Geometry check sheet. Reference: drawing and pictorial views, mm from the part's lowest x, y, z. Give positions to 0.01 mm unless a question says otherwise; leave off trailing zeros. Write each loop counter-clockwise with the first axis right and the second up, starting at its lowest first coordinate (ties: lowest second). Pieces come first, ordered by that corner, then holes. Notation, with made-up numbers: (-27.5, 67) -> (19.5, 67) arc R27 cw to (19.5, 95) -> close; hole circle Ø7 at (22.5, 71.5). An arc over 180 degrees is marked (long way). Return JSON: item names as keys, results as strings.
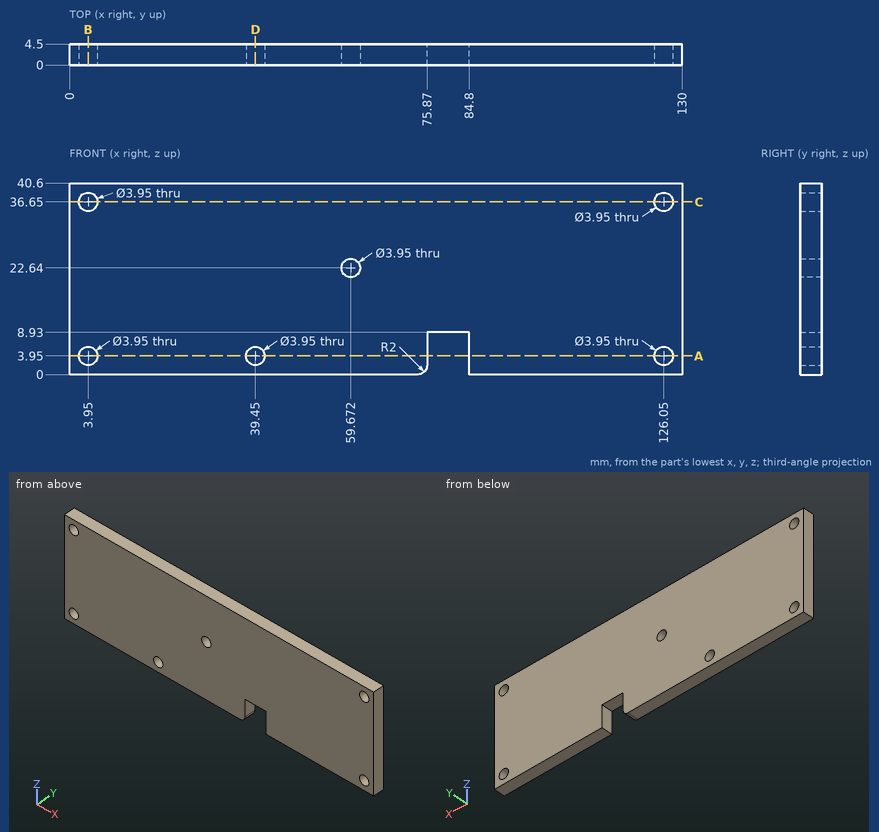
(1) Thickness scan on L1, parallel to X at y = 2.75, z = 3.95 (1 decimal); L2, parallel to X at y = 0.5, z = 5; L3, parallel to Z at x = 78, y = 2.25. Record the ranges inside material, lowest first.
Reply:
{"L1": "0 to 2, 5.9 to 37.5, 41.4 to 75.9, 84.8 to 124.1, 128 to 130", "L2": "0 to 2.28, 5.62 to 37.78, 41.12 to 75.87, 84.8 to 124.38, 127.72 to 130", "L3": "8.93 to 40.6"}
(2) Cross-section at C-C on z = 36.65. Enter the section's corners in (x, y) (1 decimal).
Reply:
{"outline": "(0, 0) -> (2, 0) -> (2, 4.5) -> (0, 4.5) -> close; (5.9, 0) -> (124.1, 0) -> (124.1, 4.5) -> (5.9, 4.5) -> close; (128, 0) -> (130, 0) -> (130, 4.5) -> (128, 4.5) -> close"}
(3) Depth check by flat-ended pin: pin 1 Ø3.5 at (x, z) = (126.05, 3.95) entering from -Y; pin 2 Ø1.3 at (x, y) = (80, 2) entering from -Z. Enter the tip coordinate at first touch or a pass-through.
Reply:
{"pin 1": "through", "pin 2": "z = 8.93"}
(4) Cross-section at B-B on x = 3.95. Enter the section's corners in (y, z) (1 decimal).
Reply:
{"outline": "(0, 0) -> (4.5, 0) -> (4.5, 2) -> (0, 2) -> close; (0, 5.9) -> (4.5, 5.9) -> (4.5, 34.7) -> (0, 34.7) -> close; (0, 38.6) -> (4.5, 38.6) -> (4.5, 40.6) -> (0, 40.6) -> close"}
(5) Cross-section at D-D on x = 39.45. Enter the section's corners in (y, z) (1 decimal), then the cut area to 3 significant figures.
Reply:
{"outline": "(0, 0) -> (4.5, 0) -> (4.5, 2) -> (0, 2) -> close; (0, 5.9) -> (4.5, 5.9) -> (4.5, 40.6) -> (0, 40.6) -> close", "area": "165 mm^2"}
(6) Cross-section at A-A on z = 3.95. Enter the section's corners in (x, y) (1 decimal).
Reply:
{"outline": "(0, 0) -> (2, 0) -> (2, 4.5) -> (0, 4.5) -> close; (5.9, 0) -> (37.5, 0) -> (37.5, 4.5) -> (5.9, 4.5) -> close; (41.4, 0) -> (75.9, 0) -> (75.9, 4.5) -> (41.4, 4.5) -> close; (84.8, 0) -> (124.1, 0) -> (124.1, 4.5) -> (84.8, 4.5) -> close; (128, 0) -> (130, 0) -> (130, 4.5) -> (128, 4.5) -> close"}
